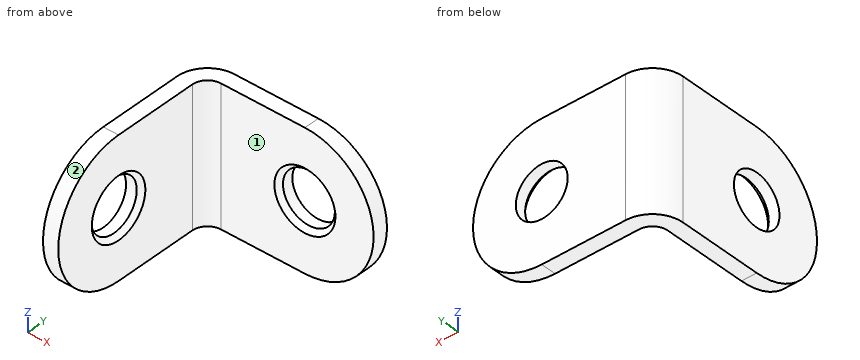
Autodesk Inventor part; units mm, degrees
ref_plane "Work Plane1" through (1, 11, 0) normal (-0.7071, -0.7071, 0) x (0, 0, -1)
ref_plane "YZ Plane" through (0, 0, 0) normal (1, 0, 0) x (0, 1, 0)
ref_plane "XZ Plane" through (0, 0, 0) normal (0, 1, 0) x (-1, 0, 0)
sketch "Sketch1" plane through (0, 0, 0) normal (0, 0, 1) x (1, 0, 0)
  line L0 (0, 0) -> (0, 12)
  line L1 (0, 12) -> (12, 12)
  line L2 (12, 12) -> (12, 11)
  line L3 (12, 11) -> (1, 11)
  line L4 (1, 11) -> (1, 0)
  line L5 (1, 0) -> (0, 0)
  dimension "d0" = 12
  dimension "d1" = 12
  dimension "d2" = 1
extrude "Extrusion1" add sketch "Sketch1" along normal blind 9
sketch "Sketch2" plane through (0, 0, 0) normal (-1, 0, 0) x (0, 0, 1)
  line L0 (9, 12) -> (9, 0)
  line L1 (0, 12) -> (9, 12)
  point P0 (0, 0)
  point P1 (4.5, 6)
  point P2 (9, 6)
  point P3 (4.5, 12)
sketch "Sketch5" plane through (1, 0, 0) normal (1, 0, 0) x (0, 0, -1)
  line L0 (0, 0) -> (0, 11)
  line L1 (0, 11) -> (-9, 11)
  line L2 (-9, 0) -> (-9, 11)
  line L3 (0, 0) -> (-9, 0)
  circle A0 centre (-4.5, 4.5) radius 4.5
  point P0 (0, 4.5)
  point P1 (-4.5, 0)
  point P2 (-9, 4.5)
hole "Hole2" at (1, 4.5, 4.5) direction (-1, 0, 0) diameter 3.4 end through all countersink diameter 4 countersink angle 90
extrude "Extrusion3" cut sketch "Sketch5" against normal blind 16.002 contours L3 A0 L0 | L3 L2 A0
ref_plane "Work Plane1" through (1, 11, 0) normal (-0.7071, -0.7071, 0) x (0, 0, -1)
mirror "Mirror1" about plane through (1, 11, 0) normal (-0.7071, -0.7071, 0) of "Extrusion3", "Hole2"
fillet "Fillet1" radius 2 1 edges at (0, 12, 4.5)
fillet "Fillet2" radius 1 1 edges at (1, 11, 4.5)
equation "\"d1\" = d0"
properties part number "Angle Bracket"
Here's how the part is built. I have some questions about the finished solid (model axes, mm). Face numbers are marked on the shaded views. A direction names the side the tool comes from. Give positions to 0.01 mm unless a question says otherwise; leave off trailing zeros. Order: outer loops, then holes, each group sorted by start corner. A loop starts at its lowest first (then second) coordinate and runs counter-clockwise, first axis right, second up. Notation, with made-up numbers: M -0.75,8.25 L 6.25,8.25 A23 cw 6.25,36.25 Z; hole C 19.25,-22.5 d11. An arc over 180 degrees is marked long. Use a Markdown table: item, result. Add a question column.
1. I need wall thicknesses on probe 1 along Z at (x, y) = (7.5, 11.6); probe 2 along X at (y, z) = (4.25, 6.75); probe 3 along X at (y, z) = (11.4, 4.5). Which ranges of each line are inside material? Lowest first, please. Write a range as from..to.
2. For pin 1 Ø1 at (x, z) = (7.5, 1.5) entering from -Y; pin 2 Ø5 at (x, z) = (2.5, 7) entering from -Y, each with a flat end and sliding along its axis, tell me the tip position at first contact or that it passes through.
3. Suppose I cut it at C-C (z = 7.25). List the corners of the cut face in (x, y) for me, and give its area (3 significant figures).
4. Suppose I cut it at A-A (z = 4.5). List the corners of the cut face in (x, y) for me, and give its area (3 significant figures).
5. On a 3-axis mill with a long thin cutter (end or side, diameter ignored), from which of +Z, -Z, +X, -X, +Y, -Y can I reach the whole of each face in a straight line? I mean the marked faces 1 and 2. Say none if no direction works.
6. Suppose I cut it at D-D (x = 3.25). List the corners of the cut face in (y, z) for me.
7. Suppose I cut it at B-B (y = 7.25). List the corners of the cut face in (x, z) for me.
Results list:
| question | item | result |
|---|---|---|
| 1 | probe 1 | z = 0..2.8, 6.2..9 |
| 1 | probe 2 | x = 0..1 |
| 1 | probe 3 | x = 0.57..5.8, 9.2..12 |
| 2 | pin 1 | stops at y = 11 |
| 2 | pin 2 | stops at y = 0.03 |
| 3 | outline | M 0,0.94 L 1,0.94 L 1,10 A1 cw 2,11 L 11.06,11 L 11.06,12 L 2,12 A2 ccw 0,10 Z |
| 3 | area | 20.5 mm² |
| 4 | outline | M 0,0 L 1,0 L 1,2.5 L 0.7,2.8 L 0,2.8 Z; M 0,6.2 L 0.7,6.2 L 1,6.5 L 1,10 A1 cw 2,11 L 5.5,11 L 5.8,11.3 L 5.8,12 L 2,12 A2 ccw 0,10 Z; M 9.2,11.3 L 9.5,11 L 12,11 L 12,12 L 9.2,12 Z |
| 4 | area | 15.4 mm² |
| 5 | face 1 | +Z, -Z, +X, -Y |
| 5 | face 2 | +X, -X, -Y |
| 6 | outline | M 11,0 L 12,0 L 12,9 L 11,9 Z |
| 7 | outline | M 0,0 L 1,0 L 1,9 L 0,9 Z |
